Part model, mm, in its own coordinate system. Face numbers are marked on the shaded views. A direction names the side the tool comes from. Give positions to 0.01 mm unless a question says otherwise; leave off trailing zeros. Write each loop counter-clockwise with the first axis right and the second up, starting at its lowest first coordinate (ties: lowest second). Pieces come first, ordered by that corner, then holes. Notation, with made-up numbers: M 42.25,-12 L 94.25,-12 A28 ccw 94.25,25 Z; hole C 83,70 d10. An arc over 180 degrees is marked long. Use a Markdown table: item, result.
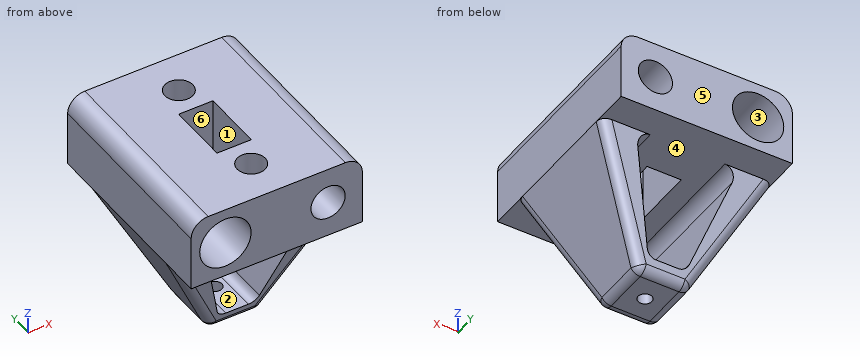
```python
from build123d import *

# Parameters (mm, degrees)
SKETCH1_W           = 50
SKETCH1_H           = 21
BOSS_EXTRUDE1_DEPTH = 58
SKETCH3_R           = 7.5
CUT_EXTRUDE1_DEPTH  = 24
CUT_EXTRUDE2_REACH  = 66.025
SKETCH4_R           = 5
CUT_EXTRUDE3_START  = -24
SKETCH5_R           = 7.5
CUT_EXTRUDE3_DEPTH  = 24
CUT_EXTRUDE4_REACH  = 66.025
SKETCH6_R           = 4.5
CUT_EXTRUDE5_REACH  = 68.558
SKETCH8_W           = 10
SKETCH8_H           = 18
BOSS_EXTRUDE3_DEPTH = 20
CUT_EXTRUDE6_DEPTH  = 37.5
CUT_EXTRUDE7_REACH  = 85.75
SKETCH13_R          = 2
SKETCH7_R           = 4.1
CUT_EXTRUDE8_DEPTH  = 15
FILLET1_R           = 5
FILLET2_R           = 3
FILLET3_R           = 3
FILLET4_R           = 3


with BuildPart() as part:
    # Sketch1 → Boss-Extrude1 (new body)
    with BuildSketch(Plane(origin=(0, 0, 0), x_dir=(1, 0, 0), z_dir=(0, 1, 0))):
        Rectangle(SKETCH1_W, SKETCH1_H)
    extrude(amount=BOSS_EXTRUDE1_DEPTH)

    # Sketch3 → Cut-Extrude1 (cut)
    with BuildSketch(Plane(origin=(0, 58, 0), x_dir=(1, 0, 0), z_dir=(0, 1, 0))):
        with Locations(Location((-15, 0, 0), (0, 0, 270))):
            Circle(SKETCH3_R)
    extrude(amount=-CUT_EXTRUDE1_DEPTH, mode=Mode.SUBTRACT)

    # Sketch4 → Cut-Extrude2 (cut, up to next)
    with BuildSketch(Plane(origin=(0, 58, 0), x_dir=(1, 0, 0), z_dir=(0, 1, 0)), mode=Mode.PRIVATE) as cut_extrude2_sk1:
        with Locations(Location((15, 0, 0), (0, 0, 270))):
            Circle(SKETCH4_R)
    cut_extrude2_tool1 = extrude(cut_extrude2_sk1.sketch, amount=-CUT_EXTRUDE2_REACH, mode=Mode.PRIVATE) & part.part
    add(cut_extrude2_tool1.solids().sort_by_distance((15, 58, 0))[0], mode=Mode.SUBTRACT)

    # Sketch5 → Cut-Extrude3 (cut)
    with BuildSketch(Plane.XZ.offset(CUT_EXTRUDE3_START)):
        with Locations(Location((-15, 0, 0), (0, 0, 90))):
            Circle(SKETCH5_R)
    extrude(amount=CUT_EXTRUDE3_DEPTH, mode=Mode.SUBTRACT)

    # Sketch6 → Cut-Extrude4 (cut, up to next)
    with BuildSketch(Plane.XZ, mode=Mode.PRIVATE) as cut_extrude4_sk1:
        with Locations(Location((-15, 0, 0), (0, 0, 270))):
            Circle(SKETCH6_R)
    cut_extrude4_tool1 = extrude(cut_extrude4_sk1.sketch, amount=-CUT_EXTRUDE4_REACH, mode=Mode.PRIVATE) & part.part
    add(cut_extrude4_tool1.solids().sort_by_distance((-15, 0, 0))[0], mode=Mode.SUBTRACT)

    # Sketch8 → Cut-Extrude5 (cut, up to next)
    with BuildSketch(Plane.XY.offset(10.5), mode=Mode.PRIVATE) as cut_extrude5_sk1:
        with Locations((0, 29)):
            Rectangle(SKETCH8_W, SKETCH8_H)
    cut_extrude5_tool1 = extrude(cut_extrude5_sk1.sketch, amount=-CUT_EXTRUDE5_REACH, mode=Mode.PRIVATE) & part.part
    add(cut_extrude5_tool1.solids().sort_by_distance((0, 29, 10.5))[0], mode=Mode.SUBTRACT)

    # Sketch11 → Boss-Extrude3 (add, symmetric)
    with BuildSketch(Plane(origin=(0, 29, 0), x_dir=(0, 0, -1), z_dir=(0, 1, 0))):
        Polygon((40.5, 5.5), (40.5, -5.5), (10.5, -15), (10.5, -25), (44.5, -7.5), (44.5, 7.5), (10.5, 25), (10.5, 15), align=None)
    extrude(amount=BOSS_EXTRUDE3_DEPTH, both=True)

    # Sketch12 → Cut-Extrude6 (cut, symmetric)
    with BuildSketch(Plane.ZY):
        Polygon((-44.5, 38), (-10.5, 49), (-44.5, 49), align=None)
        Polygon((-44.5, 20), (-10.5, 9), (-44.5, 9), align=None)
    extrude(amount=CUT_EXTRUDE6_DEPTH, both=True, mode=Mode.SUBTRACT)

    # Sketch13 → Cut-Extrude7 (cut, up to next)
    with BuildSketch(Plane(origin=(0, 0, -44.5), x_dir=(-1, 0, 0), z_dir=(0, 0, -1)), mode=Mode.PRIVATE) as cut_extrude7_sk1:
        with Locations((0, 29)):
            Circle(SKETCH13_R)
    cut_extrude7_tool1 = extrude(cut_extrude7_sk1.sketch, amount=-CUT_EXTRUDE7_REACH, mode=Mode.PRIVATE) & part.part
    add(cut_extrude7_tool1.solids().sort_by_distance((0, 29, -44.5))[0], mode=Mode.SUBTRACT)

    # Sketch7 → Cut-Extrude8 (cut)
    with BuildSketch(Plane.XY.offset(10.5)):
        with Locations((0, 46)):
            Circle(SKETCH7_R)
        with Locations(Location((0, 12, 0), (0, 0, 180))):
            Circle(SKETCH7_R)
    extrude(amount=-CUT_EXTRUDE8_DEPTH, mode=Mode.SUBTRACT)

    # Fillet1
    fillet1_edges = [part.edges().sort_by_distance(p)[0] for p in [
        (25, 29, 10.5),
        (-25, 29, 10.5),
    ]]
    fillet(fillet1_edges, radius=FILLET1_R)

    # Fillet2
    fillet2_edges = [part.edges().sort_by_distance(p)[0] for p in [
        (-7.5, 29, -44.5),
        (7.5, 29, -44.5),
        (16.25, 14.5, -27.5),
        (0, 20, -44.5),
        (-16.25, 14.5, -27.5),
        (0, 38, -44.5),
        (-16.25, 43.5, -27.5),
        (16.25, 43.5, -27.5),
    ]]
    fillet(fillet2_edges, radius=FILLET2_R)

    # Fillet3
    fillet3_edges = [part.edges().sort_by_distance(p)[0] for p in [
        (5.5, 29, -40.5),
        (-5.5, 29, -40.5),
    ]]
    fillet(fillet3_edges, radius=FILLET3_R)

    # Fillet4
    fillet4_edges = [part.edges().sort_by_distance(p)[0] for p in [
        (-15, 29, -10.5),
        (15, 29, -10.5),
    ]]
    fillet(fillet4_edges, radius=FILLET4_R)


solid = part.part
```
1. Drop flat-ended pins along their axis: P1, Ø9, axis at x = 15, z = 0, coming from the +Y side; P2, Ø13, axis at x = 0, y = 46, coming from the -Z side; P3, Ø7.5, axis at x = -13, z = 1.5, coming from the +Y side; P4, Ø5, axis at x = 0, y = 12, coming from the +Z side. Give the stop position or say it passes through.
Findings below:
| item | result |
|---|---|
| P1 | through |
| P2 | z = -10.5 |
| P3 | y = 34 |
| P4 | z = -4.5 |
2. Two-plate mould, pull along Y, no slides. Class the marked faces 4, 5 and 6: released by +Y, released by -Y, zero draft, split by the parting line, or undercut.
Findings below:
| item | result |
|---|---|
| face 4 | zero draft |
| face 5 | released by +Y |
| face 6 | undercut |
3. Cut at A-A, the plane y = 29. Give the cut face in (x, z), then the cut area to 3 significant figures.
Findings below:
| item | result |
|---|---|
| outline | M -25,-10.5 L -8.34,-42.87 A3 ccw -5.67,-44.5 L -2,-44.5 L -2,-40.5 L -3.3,-40.5 A3 cw -6.16,-38.41 L -13.76,-14.41 A3 cw -10.9,-10.5 L -5,-10.5 L -5,10.5 L -20,10.5 A5 ccw -25,5.5 Z; M 2,-44.5 L 5.67,-44.5 A3 ccw 8.34,-42.87 L 25,-10.5 L 25,5.5 A5 ccw 20,10.5 L 5,10.5 L 5,-10.5 L 10.9,-10.5 A3 cw 13.76,-14.41 L 6.16,-38.41 A3 cw 3.3,-40.5 L 2,-40.5 Z; hole C -15,0 d9; hole C 15,0 d10 |
| area | 1,170 mm2 |
4. Tool access for the marked faces 1, 2 and 3: list every direction of +Z, -Z, +X, -X, +Y, -Y with a clear straight run to the whole face (end or side of a thin tool).
Findings below:
| item | result |
|---|---|
| face 1 | +Z |
| face 2 | +Y, -Y |
| face 3 | +Y |
5. Drill centre lines: L1, parallel to X at y = 31, z = 0; L2, parallel to X at y = 43.5, z = 0; L3, parallel to Z at x = 7, y = 14.5. Where is each one in solid material? Low to high.
Findings below:
| item | result |
|---|---|
| L1 | -25 to -19.5, -10.5 to -5, 5 to 10, 20 to 25 |
| L2 | -25 to -22.5, -7.5 to -3.25, 3.25 to 10, 20 to 25 |
| L3 | -10.5 to 10.5 |
6. Cut at B-B, the plane z = 0. Give the cut face in (x, y).
Findings below:
| item | result |
|---|---|
| outline | M -25,0 L -22.5,0 L -22.5,24 L -19.5,24 L -19.5,34 L -22.5,34 L -22.5,58 L -25,58 Z; M -10.5,24 L -7.5,24 L -7.5,0 L 10,0 L 10,58 L -7.5,58 L -7.5,34 L -10.5,34 Z; M 20,0 L 25,0 L 25,58 L 20,58 Z; hole M -5,20 L 5,20 L 5,38 L -5,38 Z; hole C 0,12 d8.2; hole C 0,46 d8.2 |
7. Cut at C-C, the plane x = 0. Give the cut face in (y, z).
Findings below:
| item | result |
|---|---|
| outline | M 0,-10.5 L 20,-10.5 L 20,10.5 L 16.1,10.5 L 16.1,-4.5 L 7.9,-4.5 L 7.9,10.5 L 0,10.5 Z; M 18.71,-40.5 L 19.33,-42.42 A3 ccw 22.18,-44.5 L 27,-44.5 L 27,-40.5 Z; M 31,-44.5 L 35.82,-44.5 A3 ccw 38.67,-42.42 L 39.29,-40.5 L 31,-40.5 Z; M 38,-10.5 L 58,-10.5 L 58,10.5 L 50.1,10.5 L 50.1,-4.5 L 41.9,-4.5 L 41.9,10.5 L 38,10.5 Z |
